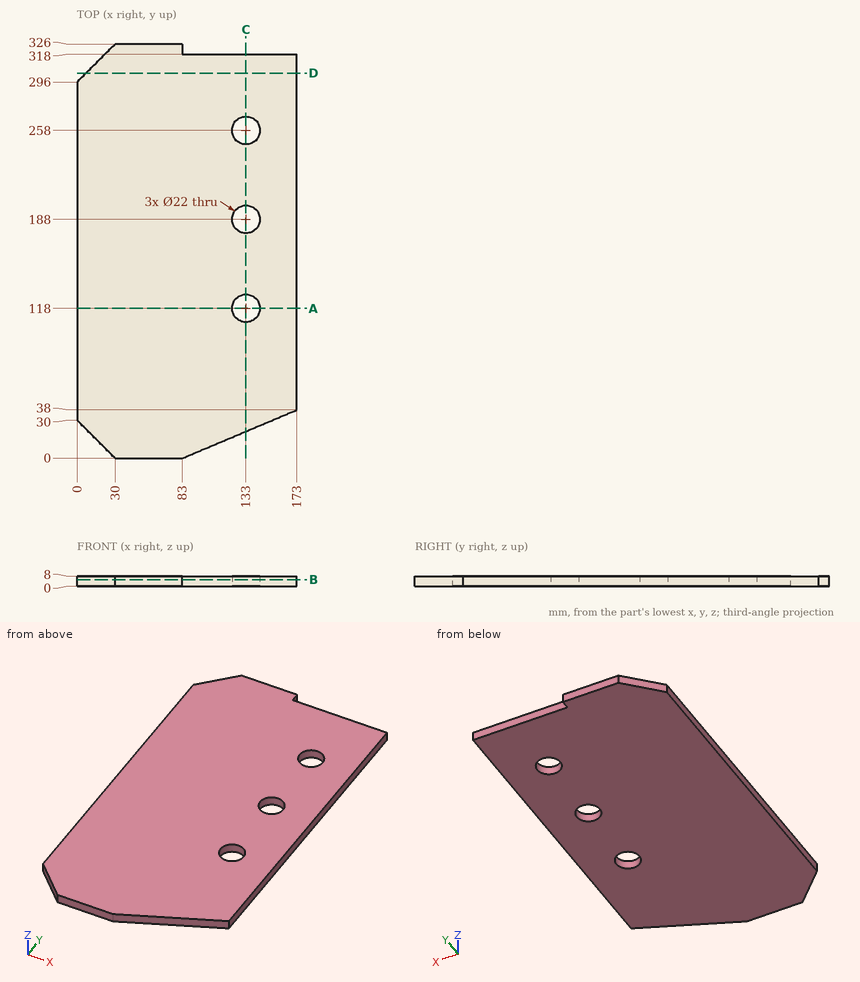
Geometry check sheet. Reference: drawing and pictorial views, mm from the part's lowest x, y, z. Round coordinates to 2 decimals unless told otherwise and drop trailing zeros. Write each loop counter-clockwise with the first axis right and the second up, starting at its lowest first coordinate (ties: lowest second). Pieces come first, ordered by that corner, then holes.
Item 1: Go/stop test with flat-tipped pins: pin 1 Ø2.5 at (x, z) = (136, 6) entering from +Y; pin 2 Ø4 at (y, z) = (322.5, 4) entering from +X; pin 3 Ø1.5 at (x, z) = (91, 3.5) entering from -Y. Record where each tip stops, or that it passes through.
Determined:
pin 1: stops at y = 318
pin 2: stops at x = 83
pin 3: stops at y = 3.06
Item 2: Section check B-B (z = 5.25). Record the boundary of the cut face in (x, y).
Determined:
outline: (0, 30) - (30, 0) - (83, 0) - (173, 38) - (173, 318) - (83, 318) - (83, 326) - (30, 326) - (0, 296) - close; hole circle Ø22 at (133, 118); hole circle Ø22 at (133, 188); hole circle Ø22 at (133, 258)
Item 3: Section check D-D (y = 303). Record the boundary of the cut face in (x, z).
Determined:
outline: (7, 0) - (173, 0) - (173, 8) - (7, 8) - close
Item 4: Section check C-C (x = 133). Record the boundary of the cut face in (y, z).
Determined:
outline: (21.11, 0) - (107, 0) - (107, 8) - (21.11, 8) - close; (129, 0) - (177, 0) - (177, 8) - (129, 8) - close; (199, 0) - (247, 0) - (247, 8) - (199, 8) - close; (269, 0) - (318, 0) - (318, 8) - (269, 8) - close
Item 5: Material ranges on line 1 along Y through (x, z) = (133, 2); line 2 along Y through (x, z) = (141.5, 1.75); line 3 along X through (y, z) = (188, 4.75), recorded low to high.
Determined:
line 1: y = 21.11 to 107, 129 to 177, 199 to 247, 269 to 318
line 2: y = 24.7 to 111.02, 124.98 to 181.02, 194.98 to 251.02, 264.98 to 318
line 3: x = 0 to 122, 144 to 173
Item 6: Section check A-A (y = 118). Record the boundary of the cut face in (x, z), plus the area to 3 significant figures.
Determined:
outline: (0, 0) - (122, 0) - (122, 8) - (0, 8) - close; (144, 0) - (173, 0) - (173, 8) - (144, 8) - close
area: 1,210 mm2
